Autodesk Inventor part; units mm, degrees
ref_plane "YZ Plane" through (0, 0, 0) normal (1, 0, 0) x (0, 1, 0)
ref_plane "XZ Plane" through (0, 0, 0) normal (0, 1, 0) x (-1, 0, 0)
ref_plane "XY Plane" through (0, 0, 0) normal (0, 0, 1) x (1, 0, 0)
sketch "Boceto1" plane through (0, 0, 0) normal (0, 0, 1) x (1, 0, 0)
  line L0 (15, -17.5) -> (15, 17.5)
  line L1 (15, 17.5) -> (-15, 17.5)
  line L2 (-15, 17.5) -> (-15, -17.5)
  line L3 (-15, -17.5) -> (-5, -17.5)
  line L4 (5, -17.5) -> (15, -17.5)
  line L5 (-4.5, -17.5) -> (-4.5, -7.5)
  line L6 (-4.5, -7.5) -> (4.5, -7.5)
  line L7 (4.5, -7.5) -> (4.5, -17.5)
  line L8 (-4.5, -17.5) -> (-5, -17.5)
  line L9 (4.5, -17.5) -> (5, -17.5)
  point P0 (0, 0)
  point P1 (15, 0)
  point P2 (0, -7.5)
  point P3 (0, -17.5)
  dimension "d0" = 30
  dimension "d1" = 35
  dimension "d7" = 10
  dimension "d8" = 9
  dimension "d9" = 15
extrude "Extrusión2" add sketch "Boceto1" along normal blind 9
sketch "Boceto2" plane through (15, -17.5, 0) normal (1, 0, 0) x (0, 0, -1)
  line L0 (0, 35) -> (0, 0)
  line L1 (0, 35) -> (-9, 35)
  line L2 (-9, 0) -> (-9, 35)
  line L3 (0, 0) -> (-9, 0)
  point P0 (0, 17.5)
  point P1 (-4.5, 5)
  dimension "d12" = 4.5
  dimension "d13" = 5
hole "Agujero1" at (15, -12.5, 4.5) direction (-1, 0, 0) diameter 5 depth 25 tip angle 118
properties part number "Tope para Motor" material "Abedul"
Design review of the part built by this model. Coordinates are the model's own, in mm. A direction names the side the tool comes from. Coordinates: 2 decimals unless noted, no trailing zeros. Order: outer loops, then holes, each group sorted by start corner. A loop starts at its lowest first (then second) coordinate and runs counter-clockwise, first axis right, second up. Notation, with made-up numbers: (-37, 89.25) -> (-14, 89.25) arc R23 ccw to (-14, 124.25) -> close; hole circle Ø9 at (74, -35.5). An arc over 180 degrees is marked (long way). One line per item, written item: value. Start each with the question number.
Q1. Insertion check: pin 1 Ø4.5 at (x, z) = (0, 3.5) entering from -Y; pin 2 Ø4 at (y, z) = (-12.5, 4.5) entering from +X. Each pin has a flat end and moves straight along its axis. Give the tip position at first contact, or say it passes through.
Q2. Take a section at C-C, the plane x = 1. State the section outline as (y, z) points, then the cut area to 3 significant figures.
Q3. Mouldability with a two-part tool opening along X and no side actions: class faces 4 (the flat face through (15, 0, 4)), 5 (the flat face through (0, 0, 0)), 6 (the flat face through (4.5, -10, 3)) as pulls with the +X half, pulls with the -X half, needs draft (parallel to the pull), parting line crosses it, or undercut.
Q4. Tool access review of faces 1 (the cylindrical face through (9.68, -10.28, 3.35)), 2 (the flat face through (0, 0, 9)), 3 (the flat face through (-4.5, -15, 3)): name each direction out of +Z, -Z, +X, -X, +Y, -Y from which nothing blocks a thin tool from reaching the whole face with its end or side.
Q5. For probe 1 along X at (y, z) = (-11, 7); probe 2 along Z at (x, y) = (11.25, -12.5); probe 3 along Y at (x, z) = (-7.45, 4.5), list the stretches that pass through material, from the lowest coordinate up.
Q6. Take a section at A-A, the plane x = -5. State the section outline as (y, z) points, then the cut area to 3 significant figures.
Q7. Take a section at B-B, the plane z = 7.75. State the section outline as (x, y) points.
Q8. Take a section at D-D, the plane y = -12. Give the number of separate pieces and of enclosed holes in the cut face, then the cut area to 3 significant figures.
Values follow:
1. pin 1: stops at y = -7.5
1. pin 2: stops at x = -10.3
2. outline: (-7.5, 0) -> (17.5, 0) -> (17.5, 9) -> (-7.5, 9) -> close
2. area: 225 mm2
3. face 4: pulls with the +X half
3. face 5: needs draft
3. face 6: undercut
4. face 1: +X
4. face 2: +Z, +X, -X, +Y, -Y
4. face 3: +Z, -Z, -Y
5. probe 1: x = -15 to -4.5, 4.5 to 15
5. probe 2: z = 0 to 2, 7 to 9
5. probe 3: y = -17.5 to -15, -10 to 17.5
6. outline: (-17.5, 0) -> (17.5, 0) -> (17.5, 9) -> (-17.5, 9) -> close; hole circle Ø5 at (-12.5, 4.5)
6. area: 295 mm2
7. outline: (-15, -17.5) -> (-4.5, -17.5) -> (-4.5, -7.5) -> (4.5, -7.5) -> (4.5, -17.5) -> (15, -17.5) -> (15, 17.5) -> (-15, 17.5) -> close
8. separate pieces: 3
8. enclosed holes: 0
8. area: 107 mm2
